Design review of the part built by this model. Coordinates are the model's own, in mm. A direction names the side the tool comes from. Give positions to 0.01 mm unless a question says otherwise; leave off trailing zeros. Loops run counter-clockwise (first coordinate to the right, second up) from the corner with the lowest first, then second, coordinate; pieces in that order, holes last. Notation, with made-up numbers: (-34, 48) -> (-24, 48) arc R28 ccw to (-24, 77) -> close; hole circle Ø2 at (33, 61.5). An arc over 180 degrees is marked (long way). Use a Markdown table: item, result. Add a question column.
1. Draft analysis for pull direction Y (two halves, no side actions). For faces 1 (the flat face through (0, -12.5, 7)), 2 (the cylindrical face through (0.007, -8.717, 17.024)), 3 (the flat face through (-7.5, -0.2, 0.5)), state which applies: pulls with the +Y half, pulls with the -Y half, needs draft (parallel to the pull), parting line crosses it, or undercut.
2. Add section C-C (z = 23). State the section outline as (x, y) points, and give its area (3 significant figures).
3. Add section B-B (y = -8.5). State the section outline as (x, z) points.
4. For pin 1 Ø12 at (y, z) = (2, 11.5) entering from -X; pin 2 Ø7.5 at (y, z) = (2, 12) entering from +X; pin 3 Ø2 at (x, y) = (3, 1) entering from +Z; pin 4 Ø8 at (x, y) = (3, 1) entering from -Z, all flat-tipped, find the tip position at first contact; note any pin that passes through.
5. Add section A-A (z = 18). State the section outline as (x, y) points.
6. For faces 4 (the flat face through (-4, 0, 1)), 5 (the flat face through (0, -8, 26)), 6 (the flat face through (4, 0, 1)), list the 3-axis set-ups (+Z, -Z, +X, -X, +Y, -Y) from which the entire face can be reached by the end or side of a thin tool; tool diameter is ignored.
7. Add section D-D (x = -1.25). State the section outline as (y, z) points, and give its area (3 significant figures).
8. To check wall thickness, follow line 1 (Z direction, x = 0, y = -8.5); line 2 (Z direction, x = 3.25, y = 9); line 3 (X direction, y = -2.25, z = 10). State the ranges of each line that lie inside material, in increasing order.
```python
from build123d import *

# Parameters (mm, degrees)
F0_W     = 15
F0_H     = 25
F1_DEPTH = 1
F2_W     = 1
F2_H     = 25
F3_DEPTH = 25
F4_R     = 1
F5_DEPTH = 1
F6_R     = 2


with BuildPart() as f1:
    # F0 (on Top) → F1 (new body)
    with BuildSketch(Plane.XY):
        Rectangle(F0_W, F0_H)
    extrude(amount=F1_DEPTH)

    # F2 (on face) → F3 (join)
    with BuildSketch(Plane.XY.offset(1)):
        Rectangle(F2_W, F2_H)
    extrude(amount=F3_DEPTH)

    # F4 (on face) → F5 (cut, through all)
    with BuildSketch(Plane.YZ.offset(0.5)):
        Polygon((-4.5, 26), (12.5, 1), (12.5, 26), align=None)
        with Locations((-8.5, 23)):
            Circle(F4_R)
        with Locations((-8.5, 18)):
            Circle(F4_R)
    extrude(amount=-F5_DEPTH, mode=Mode.SUBTRACT)

    # F6
    f6_edges = [f1.edges().sort_by_distance(p)[0] for p in [
        (0, -12.5, 26),
        (0, -4.5, 26),
    ]]
    fillet(f6_edges, radius=F6_R)


solid = f1.part
```
Taken from the geometry:
| question | item | result |
|---|---|---|
| 1 | face 1 | pulls with the -Y half |
| 1 | face 2 | undercut |
| 1 | face 3 | needs draft |
| 2 | outline | (-0.5, -12.5) -> (0.5, -12.5) -> (0.5, -9.5) -> (-0.5, -9.5) -> close; (-0.5, -7.5) -> (0.5, -7.5) -> (0.5, -2.46) -> (-0.5, -2.46) -> close |
| 2 | area | 8.04 mm^2 |
| 3 | outline | (-7.5, 0) -> (7.5, 0) -> (7.5, 1) -> (0.5, 1) -> (0.5, 17) -> (-0.5, 17) -> (-0.5, 1) -> (-7.5, 1) -> close; (-0.5, 19) -> (0.5, 19) -> (0.5, 22) -> (-0.5, 22) -> close; (-0.5, 24) -> (0.5, 24) -> (0.5, 26) -> (-0.5, 26) -> close |
| 4 | pin 1 | stops at x = -0.5 |
| 4 | pin 2 | stops at x = 0.5 |
| 4 | pin 3 | stops at z = 1 |
| 4 | pin 4 | stops at z = 0 |
| 5 | outline | (-0.5, -12.5) -> (0.5, -12.5) -> (0.5, -9.5) -> (-0.5, -9.5) -> close; (-0.5, -7.5) -> (0.5, -7.5) -> (0.5, 0.94) -> (-0.5, 0.94) -> close |
| 6 | face 4 | +Z, -X, +Y, -Y |
| 6 | face 5 | +Z, +X, -X, +Y, -Y |
| 6 | face 6 | +Z, +X, +Y, -Y |
| 7 | outline | (-12.5, 0) -> (12.5, 0) -> (12.5, 1) -> (-12.5, 1) -> close |
| 7 | area | 25.0 mm^2 |
| 8 | line 1 | z = 0 to 17, 19 to 22, 24 to 26 |
| 8 | line 2 | z = 0 to 1 |
| 8 | line 3 | x = -0.5 to 0.5 |
